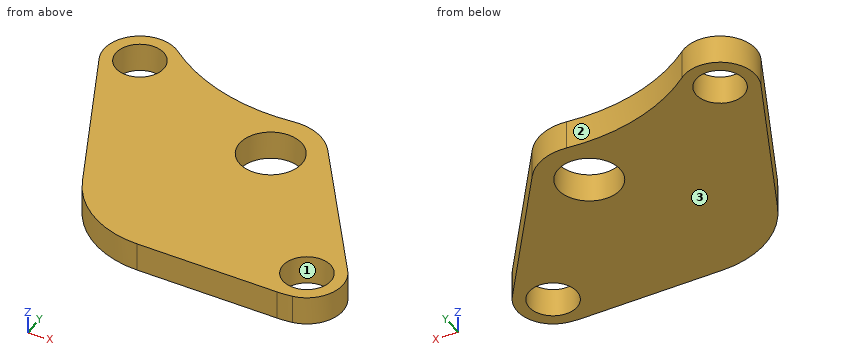
```python
from build123d import *

# Parameters (mm, degrees)
SKETCH1_R           = 2.5
SKETCH1_R_2         = 3.25
BOSS_EXTRUDE1_DEPTH = 3
FILLET1_R           = 10


with BuildPart() as part:
    # Sketch1 → Boss-Extrude1 (new body)
    with BuildSketch(Plane.XY):
        with BuildLine():
            Line((-10.17794051, -18), (10.906121257, -18))
            ThreePointArc((10.906121257, -18), (11.696957788, -17.968679831), (12.482840492, -17.874915516))
            ThreePointArc((12.482840492, -17.874915516), (15.348919612, -15.624144149), (14.949938417, -12.001825103))
            Line((14.949938417, -12.001825103), (4.279753476, 3.036604394))
            ThreePointArc((4.279753476, 3.036604394), (2.143793972, 4.789718516), (-0.586612431, 5.214704394))
            ThreePointArc((-0.586612431, 5.214704394), (-8.234060053, 5.835429339), (-15.085056175, 9.289789878))
            ThreePointArc((-15.085056175, 9.289789878), (-19.723438647, 9.258412309), (-20.782967686, 4.74255417))
            Line((-20.782967686, 4.74255417), (-10.17794051, -18))
        make_face()
        with Locations((-17.384313485, 6.327372652)):
            Circle(SKETCH1_R, mode=Mode.SUBTRACT)
        with Locations((11.891570779, -14.171822198)):
            Circle(SKETCH1_R, mode=Mode.SUBTRACT)
        Circle(SKETCH1_R_2, mode=Mode.SUBTRACT)
    extrude(amount=BOSS_EXTRUDE1_DEPTH)

    # Fillet1
    fillet1_edges = [part.edges().sort_by_distance(p)[0] for p in [
        (-10.17794051, -18, 1.5),
    ]]
    fillet(fillet1_edges, radius=FILLET1_R)


solid = part.part
```
Geometry check sheet. Reference: the model listing, model coordinates, mm. Face numbers are marked on the shaded views. Coordinates: 2 decimals unless noted, no trailing zeros. Loops run counter-clockwise (first coordinate to the right, second up) from the corner with the lowest first, then second, coordinate; pieces in that order, holes last. Notation, with made-up numbers: (-25, 78.5) -> (23, 78.5) arc R15 cw to (23, 98.5) -> close; hole circle Ø3 at (58, -12). An arc over 180 degrees is marked (long way). Put each result on its own line as item: value.
1) Cross-section at D-D on y = -10.25. Record the boundary of the cut face in (x, z).
Result set:
outline: (-13.79, 0) -> (13.71, 0) -> (13.71, 3) -> (-13.79, 3) -> close
2) Release check for a two-part mould opening along Y. For the marked faces 1, 2 and 3 record: released by +Y, released by -Y, zero draft, split by the parting line, or undercut.
Result set:
face 1: undercut
face 2: released by +Y
face 3: zero draft
3) Thickness scan on line 1 (Y direction, x = 0, z = 0.9); line 2 (Y direction, x = 14, z = 1.65); line 3 (X direction, y = -16.25, z = 0.5). Record the ranges inside material, lowest first.
Result set:
line 1: y = -18 to -3.25, 3.25 to 5.25
line 2: y = -17.27 to -15.52, -12.83 to -10.66
line 3: x = -9.46 to 10.5, 13.28 to 15.01
4) Gauge pin test, flat ends, axial feed: pin 1 Ø10.5 at (x, y) = (0, 0) entering from +Z; pin 2 Ø1 at (x, z) = (-14, 2) entering from +Y; pin 3 Ø1.5 at (y, z) = (-7, 0.5) entering from -X. Record the tip position at first contact, or that the pin passes through.
Result set:
pin 1: stops at z = 3
pin 2: stops at y = 8.85
pin 3: stops at x = -15.66
5) Cross-section at A-A on x = 0. Record the boundary of the cut face in (y, z), plus the area to 3 significant figures.
Result set:
outline: (-18, 0) -> (-3.25, 0) -> (-3.25, 3) -> (-18, 3) -> close; (3.25, 0) -> (5.25, 0) -> (5.25, 3) -> (3.25, 3) -> close
area: 50.2 mm^2
6) Cross-section at B-B on y = 0. Record the boundary of the cut face in (x, z).
Result set:
outline: (-18.57, 0) -> (-3.25, 0) -> (-3.25, 3) -> (-18.57, 3) -> close; (3.25, 0) -> (6.43, 0) -> (6.43, 3) -> (3.25, 3) -> close
7) Cross-section at C-C on z = 2.5. Record the boundary of the cut face in (x, y), plus the area to 3 significant figures.
Result set:
outline: (-20.78, 4.74) -> (-12.87, -12.23) arc R10 ccw to (-3.81, -18) -> (10.91, -18) arc R10 ccw to (12.48, -17.87) arc R3.75 ccw to (14.95, -12) -> (4.28, 3.04) arc R5.25 ccw to (-0.59, 5.21) arc R20 cw to (-15.09, 9.29) arc R3.75 ccw to start; hole circle Ø5 at (-17.38, 6.33); hole circle Ø6.5 at (0, 0); hole circle Ø5 at (11.89, -14.17)
area: 564 mm^2
